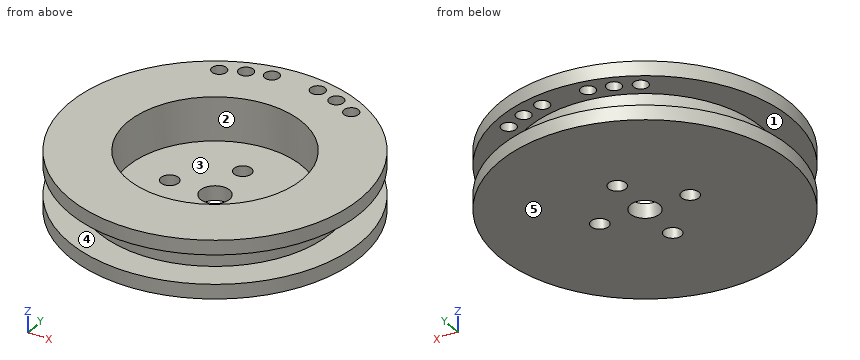
from build123d import *

# Parameters (mm, degrees)
F0_R     = 31.75
F0_R_2   = 25.4
F1_DEPTH = 3.175
F2_R     = 25.4
F3_DEPTH = 6.35
F4_R     = 31.75
F4_R_2   = 1.5875
F5_DEPTH = 3.175
F6_R     = 1.905
F6_R_2   = 3.175
F7_DEPTH = 12.7
F8_R     = 19.05
F9_DEPTH = 9.525


with BuildPart() as f1:
    # F0 (on Top) → F1 (new body)
    with BuildSketch(Plane.XY):
        Circle(F0_R)
        Circle(F0_R_2, mode=Mode.SUBTRACT)
        Circle(F0_R_2)
    extrude(amount=F1_DEPTH)

    # F2 (on face) → F3 (join)
    with BuildSketch(Plane.XY.offset(3.175)):
        Circle(F2_R)
    extrude(amount=F3_DEPTH)

    # F4 (on face) → F5 (join)
    with BuildSketch(Plane.XY.offset(9.525)):
        Circle(F4_R)
        with Locations((-14.2875, 24.746676)):
            Circle(F4_R_2, mode=Mode.SUBTRACT)
        with Locations((-9.773226, 26.851717)):
            Circle(F4_R_2, mode=Mode.SUBTRACT)
        with Locations((-4.961997, 28.140882)):
            Circle(F4_R_2, mode=Mode.SUBTRACT)
        with Locations((4.961997, 28.140882)):
            Circle(F4_R_2, mode=Mode.SUBTRACT)
        with Locations((9.773226, 26.851717)):
            Circle(F4_R_2, mode=Mode.SUBTRACT)
        with Locations((14.2875, 24.746676)):
            Circle(F4_R_2, mode=Mode.SUBTRACT)
    extrude(amount=F5_DEPTH)

    # F6 (on face) → F7 (cut, through all)
    with BuildSketch(Plane.XY.offset(12.7)):
        with Locations((0, 9.779)):
            Circle(F6_R)
        with Locations((0, -9.779)):
            Circle(F6_R)
        with Locations((-9.779, 0)):
            Circle(F6_R)
        with Locations((9.779, 0)):
            Circle(F6_R)
        Circle(F6_R_2)
    extrude(amount=-F7_DEPTH, mode=Mode.SUBTRACT)

    # F8 (on face) → F9 (cut)
    with BuildSketch(Plane.XY.offset(12.7)):
        Circle(F8_R)
    extrude(amount=-F9_DEPTH, mode=Mode.SUBTRACT)


solid = f1.part
Source: CAD feature listing. Evaluate the final solid. Frame: model axes, mm. Face numbers are marked on the shaded views. A direction names the side the tool comes from. Give positions to 0.01 mm unless a question says otherwise; leave off trailing zeros. Write each loop counter-clockwise with the first axis right and the second up, starting at its lowest first coordinate (ties: lowest second). Pieces come first, ordered by that corner, then holes. Notation, with made-up numbers: (37, 78) -> (43, 78) arc R32 ccw to (43, 115) -> close; hole circle Ø5 at (-20.75, 81). An arc over 180 degrees is marked (long way). Return JSON: item names as keys, results as strings. Group by question number.
1. Section A-A, the plane y = 0. Output: boundary loops of the cut face in (x, z) (3 decimals).
2. Material intervals for line 1 (Y direction, x = 0, z = 1.35) (3 decimals); line 2 (Y direction, x = 0.5, z = 4); line 3 (Z direction, x = 24.5, y = -8) (3 decimals), sorted ascending. Write a range as from..to.
3. Pin query (flat end, axial travel): pin 1 Ø2.5 at (x, y) = (14.29, 24.75) entering from -Z; pin 2 Ø4 at (x, z) = (3, 10) entering from +Y; pin 3 Ø2.5 at (x, y) = (0, 9.779) entering from +Z; pin 4 Ø6 at (x, y) = (9.779, 0) entering from +Z (3 decimals). Return the tip coordinate at first contact, or that it passes through.
4. Access query for the marked faces 3, 4 and 5. Directions: +Z, -Z, +X, -X, +Y, -Y. A direction counts if a zero-diameter tool reaches every point of the face in a straight line with its end or side. Return the directions, or none.
5. Section C-C, the plane z = 11.25. Count the separate pieces of the cut face and the enclosed holes in it, then the cut area to 3 significant figures.
6. Section D-D, the plane x = -15. Output: boundary loops of the cut face in (y, z) (3 decimals).
7. Mould query, pull axis X, two halves, no side actions, for the marked faces 1 and 2. Classes: +X half, -X half, draft (parallel to the pull), parting line (faces both ways), or undercut.
Determined:
{
 "1": {"outline": "(-31.75, 0) -> (-11.684, 0) -> (-11.684, 3.175) -> (-19.05, 3.175) -> (-19.05, 12.7) -> (-31.75, 12.7) -> (-31.75, 9.525) -> (-25.4, 9.525) -> (-25.4, 3.175) -> (-31.75, 3.175) -> close; (-7.874, 0) -> (-3.175, 0) -> (-3.175, 3.175) -> (-7.874, 3.175) -> close; (3.175, 0) -> (7.874, 0) -> (7.874, 3.175) -> (3.175, 3.175) -> close; (11.684, 0) -> (31.75, 0) -> (31.75, 3.175) -> (25.4, 3.175) -> (25.4, 9.525) -> (31.75, 9.525) -> (31.75, 12.7) -> (19.05, 12.7) -> (19.05, 3.175) -> (11.684, 3.175) -> close"},
 "2": {"line 1": "y = -31.75..-11.684, -7.874..-3.175, 3.175..7.874, 11.684..31.75", "line 2": "y = -25.4..-19.04, 19.04..25.4", "line 3": "z = 0..3.175, 9.525..12.7"},
 "3": {"pin 1": "stops at z = 0", "pin 2": "stops at y = 31.73", "pin 3": "passes through", "pin 4": "stops at z = 3.175"},
 "4": {"face 3": "+Z", "face 4": "none", "face 5": "-Z, +X, -X, +Y, -Y"},
 "5": {"separate pieces": "1", "enclosed holes": "7", "area": "1,980 mm2"},
 "6": {"outline": "(-27.983, 0) -> (27.983, 0) -> (27.983, 3.175) -> (20.498, 3.175) -> (20.498, 9.525) -> (23.328, 9.525) -> (23.328, 12.7) -> (11.743, 12.7) -> (11.743, 3.175) -> (-11.743, 3.175) -> (-11.743, 12.7) -> (-27.983, 12.7) -> (-27.983, 9.525) -> (-20.498, 9.525) -> (-20.498, 3.175) -> (-27.983, 3.175) -> close; (26.165, 9.525) -> (27.983, 9.525) -> (27.983, 12.7) -> (26.165, 12.7) -> close"},
 "7": {"face 1": "draft", "face 2": "undercut"}
}
